Here's how the part is built. I have some questions about the finished solid (model axes, mm). A direction names the side the tool comes from. Give positions to 0.01 mm unless a question says otherwise; leave off trailing zeros. Order: outer loops, then holes, each group sorted by start corner. A loop starts at its lowest first (then second) coordinate and runs counter-clockwise, first axis right, second up.
from build123d import *

# Parameters (mm, degrees)
SQUARE_TUBE_2_5X2_5X_188_A500_1_DEPTH = 457.2
SKETCH3_R                             = 10.3251
CUT_EXTRUDE1_DEPTH                    = 4.7752


with BuildPart() as part:
    # Sketch1 → Square tube 2.5X2.5X.188 A500(1) (new body)
    with BuildSketch(Plane.YZ):
        with BuildLine():
            Line((28.575, -31.75), (-28.575, -31.75))
            ThreePointArc((-28.575, -31.75), (-30.82006403, -30.82006403), (-31.75, -28.575))
            Line((-31.75, -28.575), (-31.75, 28.575))
            ThreePointArc((-31.75, 28.575), (-30.82006403, 30.82006403), (-28.575, 31.75))
            Line((-28.575, 31.75), (28.575, 31.75))
            ThreePointArc((28.575, 31.75), (30.82006403, 30.82006403), (31.75, 28.575))
            Line((31.75, 28.575), (31.75, -28.575))
            ThreePointArc((31.75, -28.575), (30.82006403, -30.82006403), (28.575, -31.75))
        make_face()
        with BuildLine():
            Line((24.27732, 26.9748), (-24.27732, 26.9748))
            ThreePointArc((-24.27732, 26.9748), (-26.1847264, 26.1847264), (-26.9748, 24.27732))
            Line((-26.9748, 24.27732), (-26.9748, -24.27732))
            ThreePointArc((-26.9748, -24.27732), (-26.1847264, -26.1847264), (-24.27732, -26.9748))
            Line((-24.27732, -26.9748), (24.27732, -26.9748))
            ThreePointArc((24.27732, -26.9748), (26.1847264, -26.1847264), (26.9748, -24.27732))
            Line((26.9748, -24.27732), (26.9748, 24.27732))
            ThreePointArc((26.9748, 24.27732), (26.1847264, 26.1847264), (24.27732, 26.9748))
        make_face(mode=Mode.SUBTRACT)
    extrude(amount=SQUARE_TUBE_2_5X2_5X_188_A500_1_DEPTH)

    # Sketch3 → Cut-Extrude1 (cut)
    with BuildSketch(Plane(origin=(0, 31.75, 0), x_dir=(1, 0, 0), z_dir=(0, 1, 0))):
        with Locations(Location((419.1, 0, 0), (0, 0, 270))):
            Circle(SKETCH3_R)
    extrude(amount=-CUT_EXTRUDE1_DEPTH, mode=Mode.SUBTRACT)


solid = part.part
Q1. If we section it at A-A on y = -0.5: List the corners of the cut face in (x, z) for me.
Filled sheet:
outline: (0, -31.75) - (457.2, -31.75) - (457.2, -26.97) - (0, -26.97) - close; (0, 26.97) - (457.2, 26.97) - (457.2, 31.75) - (0, 31.75) - close
Q2. For faces 4 (the face through (225, 26.975, 0)), 5 (the face through (457.2, 29, 0)), 6 (the face through (429.337, 29.396, -1.344)), which set-ups out of +Z, -Z, +X, -X, +Y, -Y let a thin tool reach every point of the face, with its end or its side?
Filled sheet:
face 4: +X, -X
face 5: +Z, -Z, +X, +Y, -Y
face 6: +Y
Q3. If we section it at B-B on z = 0: List the corners of the cut face in (x, y) for me.
Filled sheet:
outline: (0, -31.75) - (457.2, -31.75) - (457.2, -26.97) - (0, -26.97) - close; (0, 26.97) - (408.77, 26.97) - (408.77, 31.75) - (0, 31.75) - close; (429.43, 26.97) - (457.2, 26.97) - (457.2, 31.75) - (429.43, 31.75) - close
Q4. If we section it at D-D on x = 419.1: List the corners of the cut face in (y, z) for me (3 decimals).
Filled sheet:
outline: (-31.75, -28.575) arc R3.175 ccw to (-28.575, -31.75) - (28.575, -31.75) arc R3.175 ccw to (31.75, -28.575) - (31.75, -10.325) - (26.975, -10.325) - (26.975, -24.277) arc R2.697 cw to (24.277, -26.975) - (-24.277, -26.975) arc R2.697 cw to (-26.975, -24.277) - (-26.975, 24.277) arc R2.697 cw to (-24.277, 26.975) - (24.277, 26.975) arc R2.697 cw to (26.975, 24.277) - (26.975, 10.325) - (31.75, 10.325) - (31.75, 28.575) arc R3.175 ccw to (28.575, 31.75) - (-28.575, 31.75) arc R3.175 ccw to (-31.75, 28.575) - close
Q5. If we section it at C-C on x = 100: List the corners of the cut face in (y, z) for me (3 decimals).
Filled sheet:
outline: (-31.75, -28.575) arc R3.175 ccw to (-28.575, -31.75) - (28.575, -31.75) arc R3.175 ccw to (31.75, -28.575) - (31.75, 28.575) arc R3.175 ccw to (28.575, 31.75) - (-28.575, 31.75) arc R3.175 ccw to (-31.75, 28.575) - close; hole (-26.975, -24.277) arc R2.697 ccw to (-24.277, -26.975) - (24.277, -26.975) arc R2.697 ccw to (26.975, -24.277) - (26.975, 24.277) arc R2.697 ccw to (24.277, 26.975) - (-24.277, 26.975) arc R2.697 ccw to (-26.975, 24.277) - close
Q6. Thinking about a two-plate mould opening in Z: for faces 1 (the face through (225, 0, -31.75)), 2 (the face through (225, 0, 31.75)), 3 (the face through (225, -26.975, 0)), which applies, released by +Z, released by -Z, zero draft, split by the parting line, or undercut?
Filled sheet:
face 1: released by -Z
face 2: released by +Z
face 3: undercut
Q7. I need wall thicknesses on L1, parallel to Z at x = 56, y = 8; L2, parallel to X at y = 29, z = 0. Which ranges of each line are inside material? Lowest first, please.
Filled sheet:
L1: z = -31.75 to -26.97, 26.97 to 31.75
L2: x = 0 to 408.77, 429.43 to 457.2
